Autodesk Fusion 360 part; units mm, degrees
sketch "Sketch1" plane through (0, 0, 0) normal (0, 1, 0) x (1, 0, 0)
  line L0 (0, 0) -> (0, -10)
  line L1 (0, -10) -> (-2, -10)
  line L2 (-3, -13) -> (-5, -13)
  line L3 (-5, -13) -> (-5, -3)
  line L4 (-5, -3) -> (-11, -3)
  line L5 (-11, -3) -> (-11, -13)
  line L6 (-11, -13) -> (-13, -13)
  line L7 (-13, -13) -> (-13, 0)
  line L8 (-13, 0) -> (0, 0)
  line L9 (0, 0) -> (0, -4.1)
  line L10 (0, -4.1) -> (-2, -4.1)
  line L11 (-2, -4.1) -> (-2, 0)
  line L12 (-2, -10) -> (-3, -10)
  line L13 (-3, -10) -> (-3, -13)
  dimension "d1" = 10
  dimension "d2" = 2
  dimension "d3" = 4.1
  dimension "d17" = 1
  dimension "d18" = 2
  dimension "d19" = 6
  dimension "d20" = 2
  dimension "d21" = 13
  dimension "d24" = 3
  dimension "d25" = 3
  dimension "d26" = 13
revolve "Revolve1" add sketch "Sketch1" angle 360 about axis through (1.75, 0, 0) along (1, 0, 0) contours L0 L1 L2 L3 L4 L5 L6 L7 L8 L10 L11 L12 L13
sketch "Sketch2" plane through (0, 0, 0) normal (1, 0, 0) x (0, 1, 0)
  circle A0 centre (0, 0) radius 4.1
  circle A1 centre (0, 0) radius 10
  circle A2 centre (0, 0) radius 8
  circle A3 centre (0, 8) radius 1.1
  circle A4 centre (-8, 0) radius 1.1
  circle A5 centre (8, 0) radius 1.1
  circle A6 centre (0, -8) radius 1.1
  dimension "d5" = 16
  dimension "d6" = 2.2
  dimension "d7" = 2.2
  dimension "d8" = 2.2
  dimension "d9" = 2.2
extrude "Extrude1" cut sketch "Sketch2" against normal blind 20 contours A2 A5 | A2 A5 | A2 A3 | A2 A3 | A2 A6 | A2 A6 | A2 A4 | A2 A4
sketch "Sketch3" plane through (-13, 0, 0) normal (-1, 0, 0) x (0, -1, 0)
  circle A0 centre (8, 0) radius 1.1
  circle A1 centre (-8, 0) radius 1.1
  circle A2 centre (0, 8) radius 1.1
  circle A3 centre (0, -8) radius 1.1
  circle A4 centre (0, 0) radius 13
  circle A5 centre (0, 8) radius 2
  circle A6 centre (8, 0) radius 2
  circle A7 centre (0, -8) radius 2
  circle A8 centre (-8, 0) radius 2
extrude "Extrude2" cut sketch "Sketch3" against normal blind 11 contours A5 | A6 | A7 | A8
sketch "Sketch4" plane through (0, 0, 0) normal (0, 1, 0) x (1, 0, 0)
  circle A0 centre (-8, 0) radius 1
  line L0 (-5, 13) -> (-5, -13)
  dimension "d14" = 2
  dimension "d22" = 3
extrude "Extrude3" cut sketch "Sketch4" along normal through all and the other way through all
equation "d3 = ( 8.2 / 2 ) * 1 mm"
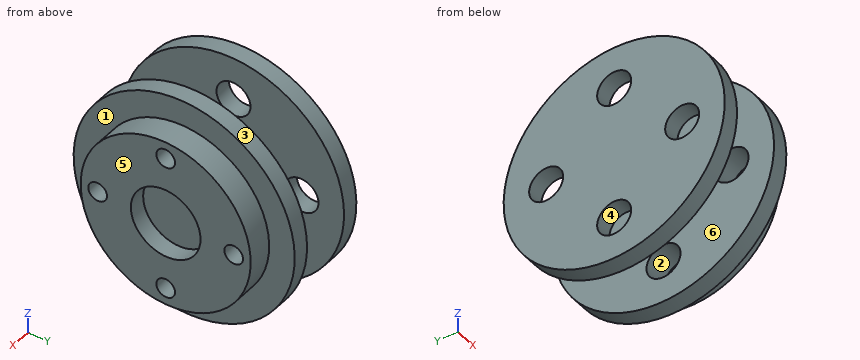
For this review, take the finished solid that the model builds, in its own axes (mm). Face numbers are marked on the shaded views. A direction names the side the tool comes from. Round coordinates to 2 decimals unless told otherwise and drop trailing zeros. Write each loop counter-clockwise with the first axis right and the second up, starting at its lowest first coordinate (ties: lowest second). Pieces come first, ordered by that corner, then holes. Notation, with made-up numbers: (-4, -14.75) -> (37, -14.75) arc R31 ccw to (37, 13.25) -> close; hole circle Ø7 at (9.25, 26). An arc over 180 degrees is marked (long way). Use one line per item in the form item = value.
1) Clearance check with flat-ended pins moving along their axes: pin 1 (1 mm diameter, centred on x = -3, y = -5.5, fed in from -Z); pin 2 (1.2 mm diameter, centred on y = 7.5, z = -0.5, fed in from -X); pin 3 (4 mm diameter, centred on x = -6.5, z = -2, fed in from -Y). State where each tip first meets the part, or that it passes through.
Found:
pin_1 = -12
pin_2 = -2
pin_3 = -12.98
2) Tool access review of the marked faces 1, 2 and 3: name each direction out of +Z, -Z, +X, -X, +Y, -Y from which nothing blocks a thin tool from reaching the whole face with its end or side.
Found:
face_1 = +X
face_2 = -X
face_3 = +X, -X
3) To check wall thickness, follow L1, parallel to Z at x = -11.95, y = 0; L2, parallel to Z at x = -1.2, y = 0; L3, parallel to X at y = 5.75, z = -9.5. State the ranges of each line that lie inside material, in increasing order. Write a range as from..to.
Found:
L1 = -13..-10, -6..6, 10..13
L2 = -10..-9.1, -6.9..-4.1, 4.1..6.9, 9.1..10
L3 = -13..-11, -5..-3
4) Mouldability with a two-part tool opening along X and no side actions: class the marked faces 4, 5 and 6 as +X half, -X half, draft (parallel to the pull), parting line (faces both ways), or undercut.
Found:
face_4 = draft
face_5 = +X half
face_6 = undercut
5) Take a section at C-C, the plane z = 8. Write out the cut boundary in (x, y).
Found:
outline = (-13, -10.25) -> (-11, -10.25) -> (-11, -2) -> (-13, -2) -> close; (-13, 2) -> (-11, 2) -> (-11, 10.25) -> (-13, 10.25) -> close; (-5, -10.25) -> (-3, -10.25) -> (-3, -6) -> (0, -6) -> (0, -1.1) -> (-2, -1.1) -> (-2, -2) -> (-5, -2) -> close; (-5, 2) -> (-2, 2) -> (-2, 1.1) -> (0, 1.1) -> (0, 6) -> (-3, 6) -> (-3, 10.25) -> (-5, 10.25) -> close
6) Take a section at A-A, the plane z = -10.5. Write out the cut boundary in (x, y), and give its area (3 significant figures).
Found:
outline = (-13, -7.66) -> (-11, -7.66) -> (-11, 7.66) -> (-13, 7.66) -> close; (-5, -7.66) -> (-3, -7.66) -> (-3, 7.66) -> (-5, 7.66) -> close
area = 61.3 mm2
7) Take a section at B-B, the plane y = 8.75. Write out the cut boundary in (x, z).
Found:
outline = (-13, -9.61) -> (-11, -9.61) -> (-11, -1.85) -> (-13, -1.85) -> close; (-13, 1.85) -> (-11, 1.85) -> (-11, 9.61) -> (-13, 9.61) -> close; (-5, -9.61) -> (-3, -9.61) -> (-3, -4.84) -> (0, -4.84) -> (0, -0.8) -> (-2, -0.8) -> (-2, -1.85) -> (-5, -1.85) -> close; (-5, 1.85) -> (-2, 1.85) -> (-2, 0.8) -> (0, 0.8) -> (0, 4.84) -> (-3, 4.84) -> (-3, 9.61) -> (-5, 9.61) -> close
8) Take a section at D-D, the plane x = -3.5. Write out the cut boundary in (y, z).
Found:
outline = circle Ø26 at (0, 0); hole circle Ø4 at (-8, 0); hole circle Ø4 at (0, -8); hole circle Ø4 at (0, 8); hole circle Ø4 at (8, 0)
